```python
from build123d import *

# Parameters (mm, degrees)
SCHIZZO1_W                   = 12
SCHIZZO1_H                   = 12
SCHIZZO1_R                   = 2.75
ESTRUSIONE_ESTRUSIONE1_DEPTH = 1
RACCORDO1_R                  = 1


with BuildPart() as part:
    # Schizzo1 → Estrusione-Estrusione1 (new body)
    with BuildSketch(Plane(origin=(0, 0, 0), x_dir=(1, 0, 0), z_dir=(0, 1, 0))):
        Rectangle(SCHIZZO1_W, SCHIZZO1_H)
        with Locations(Location((0, 0, 0), (0, 0, 270))):
            Circle(SCHIZZO1_R, mode=Mode.SUBTRACT)
    extrude(amount=ESTRUSIONE_ESTRUSIONE1_DEPTH)

    # Schizzo2 → Rivoluzione1 (revolve)
    with BuildSketch(Plane.XY, mode=Mode.PRIVATE) as rivoluzione1_sk:
        Polygon((3.75, -13), (2.75, -13), (2.75, 0), (4.748642917, 0), align=None)
    revolve(rivoluzione1_sk.sketch.rotate(Axis((0, 0, 0), (0, -1, 0)), 90), axis=Axis((0, 0, 0), (0, -1, 0)))

    # Raccordo1
    raccordo1_edges = [part.edges().sort_by_distance(p)[0] for p in [
        (0, -13, -3.75),
    ]]
    fillet(raccordo1_edges, radius=RACCORDO1_R)


solid = part.part
```
Geometry check sheet. Reference: the model listing, model coordinates, mm. A direction names the side the tool comes from. Round coordinates to 2 decimals unless told otherwise and drop trailing zeros. Loops run counter-clockwise (first coordinate to the right, second up) from the corner with the lowest first, then second, coordinate; pieces in that order, holes last. Notation, with made-up numbers: (52, 65.5) - (98, 65.5) arc R20 ccw to (98, 72.5) - close; hole circle Ø1 at (47.5, -17.75). An arc over 180 degrees is marked (long way). Use a Markdown table: item, result.
Q1. Cross-section at D-D on y = -8.5. Record the cut outline in (x, z), plus the area to 3 significant figures.
Solutions:
| item | result |
|---|---|
| outline | circle Ø8.19 at (0, 0); hole circle Ø5.5 at (0, 0) |
| area | 28.9 mm2 |
Q2. Access from +Z, -Z, +X, -X, +Y, -Y to the whole of each face (thin tool, end or side, straight path). Record for faces 1 (the flat face through (-0.1, 0.5, 6)), 2 (the flat face through (-3, 0, -4)).
Solutions:
| item | result |
|---|---|
| face 1 | +Z, +X, -X, +Y, -Y |
| face 2 | -Y |
Q3. Cross-section at A-A on z = 0. Record the cut outline in (x, y).
Solutions:
| item | result |
|---|---|
| outline | (-6, 0) - (-4.75, 0) - (-3.82, -12.08) arc R1 ccw to (-2.82, -13) - (-2.75, -13) - (-2.75, 1) - (-6, 1) - close; (2.75, -13) - (2.82, -13) arc R1 ccw to (3.82, -12.08) - (4.75, 0) - (6, 0) - (6, 1) - (2.75, 1) - close |
Q4. Go/stop test with flat-tipped pins: P1, Ø6, axis at y = -4, z = -4.5, coming from the +X side; P2, Ø1.5, axis at x = -1.5, y = -9, coming from the +Z side; P3, Ø1, axis at x = -2, y = -10, coming from the -Z side; P4, Ø5, axis at x = 0, z = 0, coming from the +Y side. Record where each tip stops, or that it passes through.
Solutions:
| item | result |
|---|---|
| P1 | stops at x = 4.21 |
| P2 | stops at z = 4 |
| P3 | stops at z = -3.69 |
| P4 | passes through |
Q5. Material ranges on line 1 (Y direction, x = 3.5, z = 3.75); line 2 (Z direction, x = -0.75, y = -10.25); line 3 (X direction, y = -5.25, z = -0.5), recorded low to high.
Solutions:
| item | result |
|---|---|
| line 1 | y = 0 to 1 |
| line 2 | z = -3.89 to -2.65, 2.65 to 3.89 |
| line 3 | x = -4.32 to -2.7, 2.7 to 4.32 |
Q6. Cross-section at C-C on y = -3.75. Record the cut outline in (x, z).
Solutions:
| item | result |
|---|---|
| outline | circle Ø8.92 at (0, 0); hole circle Ø5.5 at (0, 0) |
Q7. Cross-section at B-B on x = 0. Record the cut outline in (y, z), plus the area to 3 significant figures.
Solutions:
| item | result |
|---|---|
| outline | (-13, -2.82) arc R1 ccw to (-12.08, -3.82) - (0, -4.75) - (0, -6) - (1, -6) - (1, -2.75) - (-13, -2.75) - close; (-13, 2.75) - (1, 2.75) - (1, 6) - (0, 6) - (0, 4.75) - (-12.08, 3.82) arc R1 ccw to (-13, 2.82) - close |
| area | 45.1 mm2 |
